```python
from build123d import *

# Parameters (mm, degrees)
F0_W        = 40
F0_H        = 40
F1_DEPTH    = 600
F3_T1_DEPTH = 247.8831037137
F4_R        = 3
F6_DEPTH    = 12
F5_R        = 3
F7_DEPTH    = 12
F8_R        = 5
F9_DEPTH    = 12


# Not quite as in the source:
# - a fillet or chamfer that OpenCascade refuses, or shapes differently, is made with other operations: its cross-section is extruded or revolved along the edge and cut away or added
# - a feature of the source that left no trace in its solid (it failed there, or was rolled back) is left out


with BuildPart() as f1:
    # F0 (on Top) → F1 (new body)
    with BuildSketch(Plane.XY):
        with Locations((20, 20)):
            Rectangle(F0_W, F0_H)
    extrude(amount=F1_DEPTH)

    # F3: chamfer of 40 x 7.0530792283 on 2 edges, made by hand

    # F3_s2 → F3_t1 (cut)
    with BuildSketch(Plane.YZ.offset(-103.9415518568)):
        Polygon((40, 7.0530792283), (0, 0), (40, 0), align=None)
        Polygon((0, 592.9469207717), (40, 600), (0, 600), align=None)
    extrude(amount=F3_T1_DEPTH, mode=Mode.SUBTRACT)

    # F4 (on face) → F6 (cut)
    with BuildSketch(Plane.XZ):
        with Locations((15, 562.9469207717)):
            Circle(F4_R)
    extrude(amount=-F6_DEPTH, mode=Mode.SUBTRACT)

    # F5 (on face) → F7 (cut)
    with BuildSketch(Plane.YZ.offset(40)):
        with Locations((25, 566.8922969328)):
            Circle(F5_R)
    extrude(amount=-F7_DEPTH, mode=Mode.SUBTRACT)

    # F8 (on face) → F9 (cut)
    with BuildSketch(Plane(origin=(0, -101.3998954134, 575.0673833693), x_dir=(1, 0, 0), z_dir=(0, -0.1736481777, 0.984807753))):
        with Locations((20.0023799473, 122.9641521036)):
            Circle(F8_R)
    extrude(amount=-F9_DEPTH, mode=Mode.SUBTRACT)


solid = f1.part
```
Part model, mm, in its own coordinate system. Round coordinates to 2 decimals unless told otherwise and drop trailing zeros.
Item 1: Drop flat-ended pins along their axis: P1, Ø12, axis at x = 34.5, z = 516.5, coming from the -Y side; P2, Ø3, axis at x = 16, y = 18.5, coming from the +Z side; P3, Ø2, axis at x = 34.5, y = 5.5, coming from the -Z side; P4, Ø8, axis at x = 17.5, y = 26.5, coming from the +Z side. Give the stop position or say it passes through.
Item 2: Mould opens along Z. For faces 1 (the face through (19.932, 21.849, 584.614)), 2 (the face through (0, 20, 296)), 3 (the face through (15.28, 15.28, 595.64)) say: +Z half, -Z half, draft (parallel to the pull), parting line (faces both ways), or undercut.
Item 3: Drill centre lines: line 1 (Z direction, x = 35, y = 25); line 2 (Z direction, x = 30.5, y = 23.5); line 3 (Z direction, x = 8, y = 2). Where is each one in solid material? Low to high.
A:
1. P1: stops at y = 0
1. P2: stops at z = 596.41
1. P3: stops at z = 0.79
1. P4: stops at z = 598.32
2. face 1: undercut
2. face 2: draft
2. face 3: +Z half
3. line 1: z = 4.41 to 563.89, 569.89 to 597.36
3. line 2: z = 4.14 to 564.29, 569.49 to 597.09
3. line 3: z = 0.35 to 593.3
